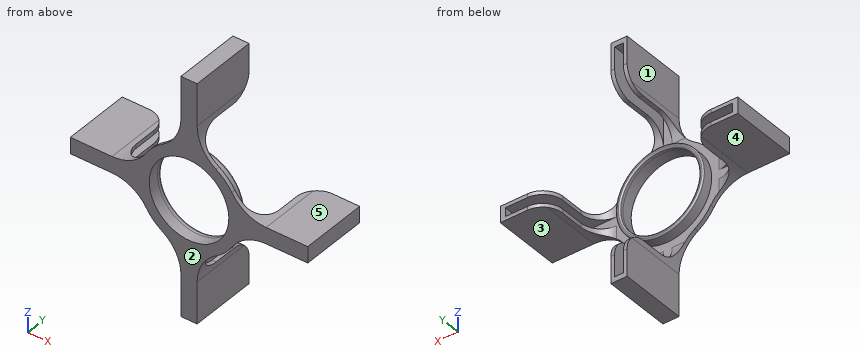
```python
from build123d import *

# Parameters (mm, degrees)
SKETCH1_R                = 37.5
BASE_DEPTH               = 3
SKETCH2_W                = 12
SKETCH2_H                = 88
FIN_EXTENSION_BASE_DEPTH = 3
FIN_CRADDLE_DEPTH        = 50
FILLET2_R                = 30
FILLET1_R                = 15
CIRPATTERN1_COUNT        = 4
FILLET2_OF_CIRPATTERN1_R = 30
FILLET1_OF_CIRPATTERN1_R = 15
BOSS_EXTRUDE5_REACH      = 132.419
SKETCH4_R                = 32.5
SKETCH4_R_2              = 29.5
FILLET3_R                = 5
FILLET4_R                = 1
SKETCH5_R                = 29.5
CUT_EXTRUDE1_DEPTH       = 135.119349872


with BuildPart() as part:
    # Sketch1 → BASE (new body)
    with BuildSketch(Plane(origin=(0, 0, 0), x_dir=(1, 0, 0), z_dir=(0, 1, 0))):
        with Locations(Location((0, 0, 0), (0, 0, 270))):
            Circle(SKETCH1_R)
    extrude(amount=BASE_DEPTH)

    # Sketch2 → FIN EXTENSION BASE (add)
    with BuildSketch(Plane(origin=(0, 0, 0), x_dir=(1, 0, 0), z_dir=(0, 1, 0))):
        with Locations((0, 44)):
            Rectangle(SKETCH2_W, SKETCH2_H)
    fin_extension_base = extrude(amount=FIN_EXTENSION_BASE_DEPTH)

    # Sketch3 → FIN CRADDLE (add)
    with BuildSketch(Plane(origin=(0, 0, 0), x_dir=(1, 0, 0), z_dir=(0, 1, 0))):
        Polygon((-6, 53), (-3.25, 53), (-3.25, 84.25), (3.25, 84.25), (3.25, 53), (6, 53), (6, 88), (-6, 88), align=None)
    fin_craddle = extrude(amount=FIN_CRADDLE_DEPTH)

    # Fillet2
    fillet2_edges = [part.edges().sort_by_distance(p)[0] for p in [
        (6, 1.5, -37.016888038),
        (-6, 1.5, -37.016888038),
    ]]
    fillet(fillet2_edges, radius=FILLET2_R)

    # Fillet1
    fillet1_edges = [part.edges().sort_by_distance(p)[0] for p in [
        (-4.765646996, 50, -53),
        (4.765646996, 50, -53),
        (-4.765646996, 3, -53),
        (4.765646996, 3, -53),
    ]]
    fillet(fillet1_edges, radius=FILLET1_R)

    # CirPattern1: FIN EXTENSION BASE, FIN CRADDLE ×4 about axis
    cirpattern1_axis = Axis((0, 0, 0), (0, 1, 0))
    add([fin_extension_base.rotate(cirpattern1_axis, i * 360 / CIRPATTERN1_COUNT) for i in range(1, CIRPATTERN1_COUNT)])
    add([fin_craddle.rotate(cirpattern1_axis, i * 360 / CIRPATTERN1_COUNT) for i in range(1, CIRPATTERN1_COUNT)])

    # Fillet2 of CirPattern1
    fillet2_of_cirpattern1_edges = [part.edges().sort_by_distance(p)[0] for p in [
        (-37.016888038, 1.5, -6),
        (-37.016888038, 1.5, 6),
        (-6, 1.5, 37.016888038),
        (6, 1.5, 37.016888038),
        (37.016888038, 1.5, 6),
        (37.016888038, 1.5, -6),
    ]]
    fillet(fillet2_of_cirpattern1_edges, radius=FILLET2_OF_CIRPATTERN1_R)

    # Fillet1 of CirPattern1
    fillet1_of_cirpattern1_edges = [part.edges().sort_by_distance(p)[0] for p in [
        (-53, 50, 4.765646996),
        (-53, 50, -4.765646996),
        (-53, 3, 4.765646996),
        (-53, 3, -4.765646996),
        (4.765646996, 50, 53),
        (-4.765646996, 50, 53),
        (4.765646996, 3, 53),
        (-4.765646996, 3, 53),
        (53, 50, -4.765646996),
        (53, 50, 4.765646996),
        (53, 3, -4.765646996),
        (53, 3, 4.765646996),
    ]]
    fillet(fillet1_of_cirpattern1_edges, radius=FILLET1_OF_CIRPATTERN1_R)

    # Sketch4 → Boss-Extrude5 (add, up to next)
    with BuildSketch(Plane(origin=(0, 11, 0), x_dir=(1, 0, 0), z_dir=(0, 1, 0)), mode=Mode.PRIVATE) as boss_extrude5_sk1:
        with Locations(Location((0, 0, 0), (0, 0, 270))):
            Circle(SKETCH4_R)
        with Locations(Location((0, 0, 0), (0, 0, 270))):
            Circle(SKETCH4_R_2, mode=Mode.SUBTRACT)
    boss_extrude5_tool1 = extrude(boss_extrude5_sk1.sketch, amount=-BOSS_EXTRUDE5_REACH, mode=Mode.PRIVATE) - part.part
    add(boss_extrude5_tool1.solids().sort_by_distance((0, 11, -31.580761))[0])

    # Fillet3
    fillet3_edges = [part.edges().sort_by_distance(p)[0] for p in [
        (0, 3, -29.5),
    ]]
    fillet(fillet3_edges, radius=FILLET3_R)

    # Fillet4
    fillet4_edges = [part.edges().sort_by_distance(p)[0] for p in [
        (0, 11, -32.5),
        (0, 11, -29.5),
    ]]
    fillet(fillet4_edges, radius=FILLET4_R)

    # Sketch5 → Cut-Extrude1 (cut, through all)
    with BuildSketch(Plane(origin=(0, 0, 0), x_dir=(1, 0, 0), z_dir=(0, 1, 0))):
        with Locations(Location((0, 0, 0), (0, 0, 270))):
            Circle(SKETCH5_R)
    extrude(amount=CUT_EXTRUDE1_DEPTH, mode=Mode.SUBTRACT)


solid = part.part
```
Part model, mm, in its own coordinate system. Face numbers are marked on the shaded views. A direction names the side the tool comes from. Round coordinates to 2 decimals unless told otherwise and drop trailing zeros. Write each loop counter-clockwise with the first axis right and the second up, starting at its lowest first coordinate (ties: lowest second). Pieces come first, ordered by that corner, then holes.
Item 1: Probe L1, parallel to X at y = 5.75, z = 0; L2, parallel to X at y = 26, z = 65.5. List the from-to ranges inside material, lowest first.
Results:
L1: x = -88 to -84.25, -32.5 to -29.5, 29.5 to 32.5, 84.25 to 88
L2: x = -6 to -3.25, 3.25 to 6
Item 2: Cut at C-C, the plane y = 30. Count the separate pieces of the cut face and the enclosed holes in it, plus the area to 3 significant figures.
Results:
separate pieces: 4
enclosed holes: 0
area: 871 mm2
Item 3: Which spindle directions (+Z, -Z, +X, -X, +Y, -Y) get a long thin tool onto all of the face, cutting with end or side? Do the marked faces 1, 2, 3, 4 and 5. Say none if no direction does.
Results:
face 1: +Z, -X, +Y, -Y
face 2: +Z, -Z, +X, -X, -Y
face 3: -Z, +X, +Y, -Y
face 4: -Z, -X, +Y, -Y
face 5: +Z, +X, +Y, -Y
Item 4: Cut at B-B, the plane z = 0. Give the cut face in (x, y).
Results:
outline: (-88, 0) - (-29.5, 0) - (-29.5, 10) arc R1 ccw to (-30.5, 11) - (-31.5, 11) arc R1 ccw to (-32.5, 10) - (-32.5, 3) - (-84.25, 3) - (-84.25, 50) - (-88, 50) - close; (29.5, 0) - (88, 0) - (88, 50) - (84.25, 50) - (84.25, 3) - (32.5, 3) - (32.5, 10) arc R1 ccw to (31.5, 11) - (30.5, 11) arc R1 ccw to (29.5, 10) - close
Item 5: Cut at A-A, the plane x = 0. Give the cut face in (y, z).
Results:
outline: (0, -88) - (50, -88) - (50, -84.25) - (3, -84.25) - (3, -32.5) - (10, -32.5) arc R1 ccw to (11, -31.5) - (11, -30.5) arc R1 ccw to (10, -29.5) - (0, -29.5) - close; (0, 29.5) - (10, 29.5) arc R1 ccw to (11, 30.5) - (11, 31.5) arc R1 ccw to (10, 32.5) - (3, 32.5) - (3, 84.25) - (50, 84.25) - (50, 88) - (0, 88) - close
Item 6: Drop flat-ended pins along their axis: pin 1 Ø24.5 at (y, z) = (27.5, 78.5) entering from -X; pin 2 Ø15.5 at (x, y) = (-80, 37) entering from -Z; pin 3 Ø24.5 at (y, z) = (31.5, 74.5) entering from +X. Give the stop position or say it passes through.
Results:
pin 1: stops at x = -6
pin 2: stops at z = -6
pin 3: stops at x = 6
